Geometry check sheet. Reference: the model listing, model coordinates, mm. Coordinates: 2 decimals unless noted, no trailing zeros. Loops run counter-clockwise (first coordinate to the right, second up) from the corner with the lowest first, then second, coordinate; pieces in that order, holes last. Notation, with made-up numbers: (76.5, 63) - (87.5, 63) arc R34 ccw to (87.5, 94) - close; hole circle Ø3 at (47, 51). An arc over 180 degrees is marked (long way). Write each question's results on one line, items separated by ' | '. Start each with the question number.
(1) Go/stop test with a flat-tipped pin: pin 1 Ø3 at (x, y) = (-44.5, 17.5) entering from -Z. Record where the tip stops, or that it passes through.
(2) Sectioned sample at B-B (y = 65.5). Enter the section's corners in (x, z).
(3) Sectioned sample at A-A (y = -43.5). Enter the section's corners in (x, z), plus the area to 3 significant figures.
(4) Material ranges on probe 1 along Y at (x, z) = (-40, 3.25); probe 2 along Y at (x, z) = (40, 1.25); probe 3 along X at (y, z) = (73, 1.9), recorded low to high.
Autodesk Inventor part; units mm, degrees
ref_plane "YZ Plane" through (0, 0, 0) normal (1, 0, 0) x (0, 1, 0)
ref_plane "XZ Plane" through (0, 0, 0) normal (0, 1, 0) x (-1, 0, 0)
ref_plane "XY Plane" through (0, 0, 0) normal (0, 0, 1) x (1, 0, 0)
sketch "Sketch1" plane through (0, 0, 0) normal (0, 0, 1) x (1, 0, 0)
  line L0 (-150, -80) -> (40, -80)
  line L1 (150, -80) -> (150, 80) construction
  line L2 (40, 80) -> (-150, 80)
  line L3 (-150, 80) -> (-150, -80)
  line L4 (-150, -80) -> (150, 80) construction
  line L5 (150, -80) -> (-150, 80) construction
  line L6 (-150, 0) -> (-107, 0) construction
  line L7 (-107, 0) -> (33.79, 0) construction
  line L8 (-7.3128, 0) -> (74.6872, 0) construction
  line L9 (33.6872, 41) -> (74.6872, 41) construction
  line L10 (74.6872, 41) -> (74.6872, 0) construction
  circle A0 centre (74.6872, 41) radius 2 construction
  circle A1 centre (74.6872, -41) radius 2 construction
  circle A2 centre (-7.3128, 41) radius 2 construction
  circle A3 centre (-7.3128, -41) radius 2 construction
  line L11 (150, 0) -> (120, 0) construction
  line L12 (120, 0) -> (120, 0)
  arc A4 (40, -80) -> (120, 0) centre (40, 0) ccw
  arc A5 (120, 0) -> (40, 80) centre (40, 0) ccw
  line L13 (120, 0) -> (115, 0) construction
  circle A6 centre (115, 0) radius 1.5
  line L14 (40, 0) -> (111.7631, 71.7631) construction
  line L15 (96.5685, -56.5685) -> (93.033, -53.033) construction
  circle A7 centre (93.033, -53.033) radius 1.5
  line L16 (40, -80) -> (40, -75) construction
  circle A8 centre (40, -75) radius 1.5
  line L17 (40, -75) -> (-15, -75) construction
  line L18 (-15, -75) -> (-70, -75) construction
  line L19 (-150, -75) -> (-145, -75) construction
  circle A9 centre (-15, -75) radius 1.5
  circle A10 centre (-70, -75) radius 1.5
  circle A11 centre (-145, -75) radius 1.5
  circle A12 centre (-145, 0) radius 1.5
  circle A13 centre (93.033, 53.033) radius 1.5
  circle A14 centre (40, 75) radius 1.5
  circle A15 centre (-15, 75) radius 1.5
  circle A16 centre (-70, 75) radius 1.5
  circle A17 centre (-145, 75) radius 1.5
  line L20 (-145, -80) -> (-145, -75) construction
  line L21 (-150, 0) -> (-145, 0)
  line L22 (120, 0) -> (105, 0) construction
  line L23 (105, -30) -> (105, 30) construction
  circle A18 centre (105, -30) radius 4 construction
  circle A19 centre (105, 30) radius 4 construction
  circle A20 centre (105, -30) radius 1.5
  circle A21 centre (105, 30) radius 1.5
  line L24 (105, 0) -> (55, 0) construction
  line L25 (55, -70) -> (55, 70) construction
  circle A22 centre (55, -70) radius 1.5
  circle A23 centre (55, -70) radius 4 construction
  line L26 (-150, 0) -> (-135, 0) construction
  line L27 (-135, -72.5) -> (-135, 72.5) construction
  circle A24 centre (-135, -72.5) radius 1.5
  circle A25 centre (-135, -72.5) radius 4 construction
  line L28 (-135, 0) -> (-40, 0) construction
  line L29 (-40, -72.5) -> (-40, 72.5) construction
  circle A26 centre (-40, -72.5) radius 4 construction
  circle A27 centre (-40, -72.5) radius 1.5
  circle A28 centre (55, 70) radius 1.5
  circle A29 centre (55, 70) radius 4 construction
  circle A30 centre (-135, 72.5) radius 1.5
  circle A31 centre (-135, 72.5) radius 4 construction
  circle A32 centre (-40, 72.5) radius 4 construction
  circle A33 centre (-40, 72.5) radius 1.5
  line L30 (-150, 60) -> (-120, 60) construction
  line L31 (-120, 80) -> (-120, 60) construction
  circle A34 centre (-120, 60) radius 1.75
  circle A35 centre (-118.73, 11.74) radius 1.75
  line L32 (-120, 60) -> (-67.93, 60) construction
  line L33 (-150, 11.74) -> (-118.73, 11.74) construction
  line L34 (-118.73, 60) -> (-118.73, 11.74) construction
  line L35 (-67.93, 60) -> (-67.93, 54.92) construction
  circle A36 centre (-67.93, 54.92) radius 1.75
  line L36 (-67.93, 54.92) -> (-67.93, 26.98) construction
  circle A37 centre (-67.93, 26.98) radius 1.75
  point P0 (0, 0)
  point P1 (120, -80)
  point P2 (120, 0)
  dimension "d0" = 300
  dimension "d1" = 160
  dimension "d4" = 43
  dimension "d6" = 140.79
  dimension "d9" = 82
  dimension "d11" = 4
  dimension "d47" = 30
  dimension "d49" = 80
  dimension "LF" = 5
  dimension "Furos" = 3
  dimension "d52" = 45
  dimension "d53" = 5
  dimension "d55" = 3
  dimension "d56" = 5
  dimension "d57" = 3
  dimension "d58" = 55
  dimension "d59" = 55
  dimension "d60" = 5
  dimension "d61" = 3
  dimension "d62" = 3
  dimension "d63" = 3
  dimension "d64" = 3
  dimension "d65" = 5
  dimension "d66" = 5
  dimension "d67" = 15
  dimension "d68" = 60
  dimension "d69" = 8
  dimension "d70" = 8
  dimension "d71" = 3
  dimension "FA" = 3
  dimension "d73" = 50
  dimension "d74" = 140
  dimension "d75" = 3
  dimension "AA" = 8
  dimension "d77" = 15
  dimension "d78" = 145
  dimension "d79" = 3
  dimension "d80" = 8
  dimension "d81" = 95
  dimension "d82" = 145
  dimension "d83" = 8
  dimension "d84" = 3
  dimension "d85" = 30
  dimension "d86" = 20
  dimension "d87" = 3.5
  dimension "d89" = 3.5
  dimension "d90" = 52.07
  dimension "d94" = 31.27
  dimension "d95" = 48.26
  dimension "d96" = 5.08
  dimension "d97" = 3.5
  dimension "d98" = 27.94
  dimension "d99" = 3.5
  dimension "d100" = 41
  dimension "d101" = 41
  dimension "d103" = 74.6872
  dimension "d104" = 82
  dimension "d105" = 41
extrude "Extrusion1" add sketch "Sketch1" along normal blind 4
fillet "Fillet1" radius 5 2 edges at (-150, -80, 2) (-150, 80, 2)
equation "\"d9\" = L_furos"
equation "\"d53\" = LF"
equation "\"d55\" = Furos"
equation "\"d56\" = LF"
equation "\"d57\" = Furos"
equation "\"d60\" = LF"
equation "\"d61\" = Furos"
equation "\"d62\" = Furos"
equation "\"d63\" = Furos"
equation "\"d64\" = Furos"
equation "\"d65\" = LF"
equation "\"d66\" = LF"
equation "\"d69\" = AA"
equation "\"d70\" = AA"
equation "\"d71\" = FA"
equation "\"d75\" = FA"
equation "\"d79\" = FA"
equation "\"d80\" = AA"
equation "\"d83\" = AA"
equation "\"d84\" = FA"
properties part number "Base_solida_Down_test"
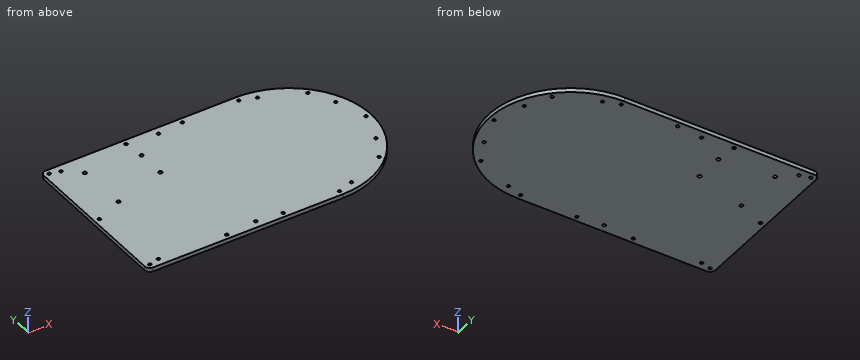
Outcome:
1) pin 1: stops at z = 0
2) outline: (-150, 0) - (85.93, 0) - (85.93, 4) - (-150, 4) - close
3) outline: (-150, 0) - (107.14, 0) - (107.14, 4) - (-150, 4) - close | area: 1,030 mm2
4) probe 1: y = -80 to -74, -71 to 71, 74 to 80 | probe 2: y = -80 to -76.5, -73.5 to 73.5, 76.5 to 80 | probe 3: x = -150 to -136.41, -133.59 to -41.41, -38.59 to 72.73
